Read the model definition and answer for the solid it produces. Units are mm, in the model's axes. Face numbers are marked on the shaded views. A direction names the side the tool comes from. Round coordinates to 2 decimals unless told otherwise and drop trailing zeros. Write each loop counter-clockwise with the first axis right and the second up, starting at its lowest first coordinate (ties: lowest second). Pieces come first, ordered by that corner, then holes. Notation, with made-up numbers: (43.5, 10.25) - (57.5, 10.25) arc R16 ccw to (57.5, 34.25) - close; hole circle Ø7 at (9, -5.75). An arc over 180 degrees is marked (long way). Answer as CSV lines item,"result". Start each with the question number.
1) Which of the six approach directions +Z, -Z, +X, -X, +Y, -Y give full straight-line access (tool end or side, diameter ignored) to the marked faces 1, 2 and 3?
2) Find section A-A on x = 9.5. Determine the outline of the cut face in (y, z).
3) For a pull along Y with two mould halves and no side action, classify the marked faces 4, 5, 6 and 7 as +Y half, -Y half, draft (parallel to the pull), parting line (faces both ways), or undercut.
4) Each of these flat-tipped pins is pushed along its axis until it touches: pin 1 (1.5 mm diameter, centred on y = -20.5, z = 6, fed in from -X); pin 2 (5 mm diameter, centred on x = 6, z = 4, fed in from -Y); pin 3 (5 mm diameter, centred on y = -37.5, z = 4.5, fed in from -X). Where does it stop, or does it pass through?
5) Find section B-B on z = 6.25. Determine the outline of the cut face in (x, y).
6) Find section D-D on y = -27.5. Determine the outline of the cut face in (x, z), then the cut area to 3 significant figures.
7) Consider line 1 along Y through (x, z) = (11, 2.25); line 2 along Y through (x, z) = (13, 7.25); line 3 along Y through (x, z) = (14.75, 2.75). Determine where each line is inside the solid, lowest interval first.
8) Find section C-C on x = 6.5. Determine the outline of the cut face in (y, z).
from build123d import *

# Parameters (mm, degrees)
F1_DEPTH = 10
F2_R     = 1
F3_SIZE  = 0.99999


# Not quite as in the source:
# - a fillet or chamfer is up to 0.001 mm smaller than in the source, because OpenCascade refuses the exact size


with BuildPart() as f1:
    # F0 (on Top) → F1 (new body)
    with BuildSketch(Plane.XY):
        Polygon((18, 0), (0, 0), (0, -3), (15, -3), (15, -13), (13, -15), (15, -17), (15, -37), (12, -37), (12, -34), (9, -34), (9, -40), (18, -40), align=None)
    extrude(amount=F1_DEPTH)

    # F2
    f2_edges = [f1.edges().sort_by_distance(p)[0] for p in [
        (13, -15, 5),
        (15, -13, 5),
        (15, -37, 5),
        (15, -17, 5),
        (15, -3, 5),
        (12, -37, 5),
    ]]
    fillet(f2_edges, radius=F2_R)

    # F3 (size 1 in the source; OpenCascade refuses exactly that, so slightly less here)
    f3_edges = [f1.edges().sort_by_distance(p)[0] for p in [
        (7, -3, 10),
        (14.707107, -3.292893, 10),
        (0, -1.5, 10),
        (15, -8.292893, 10),
        (9, 0, 10),
        (14.92388, -12.96847, 10),
        (18, -20, 10),
        (14.207107, -13.792893, 10),
        (13.5, -40, 10),
        (13.414214, -15, 10),
        (9, -37, 10),
        (14.207107, -16.207107, 10),
        (10.5, -34, 10),
        (14.92388, -17.03153, 10),
        (12, -35, 10),
        (15, -26.707107, 10),
        (12.292893, -36.707107, 10),
        (14.707107, -36.707107, 10),
        (13.5, -37, 10),
        (7, -3, 0),
        (14.707107, -3.292893, 0),
        (0, -1.5, 0),
        (15, -8.292893, 0),
        (9, 0, 0),
        (14.92388, -12.96847, 0),
        (18, -20, 0),
        (14.207107, -13.792893, 0),
        (13.5, -40, 0),
        (13.414214, -15, 0),
        (9, -37, 0),
        (14.207107, -16.207107, 0),
        (10.5, -34, 0),
        (14.92388, -17.03153, 0),
        (12, -35, 0),
        (15, -26.707107, 0),
        (12.292893, -36.707107, 0),
        (14.707107, -36.707107, 0),
        (13.5, -37, 0),
    ]]
    chamfer(f3_edges, length=F3_SIZE)


solid = f1.part
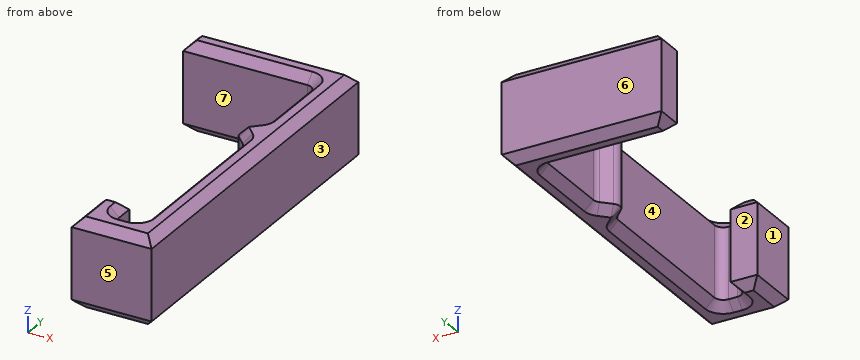
Check values:
1,face 1,"+Z, -Z, -X, -Y"
1,face 2,"+Z, -Z, -X"
1,face 3,"+Z, -Z, +X, +Y, -Y"
2,outline,"(-40, 1) - (-39.5, 0.5) - (-34.5, 0.5) - (-34, 1) - (-34, 9) - (-34.5, 9.5) - (-39.5, 9.5) - (-40, 9) - close; (-3, 1) - (-2, 0) - (-1, 0) - (0, 1) - (0, 9) - (-1, 10) - (-2, 10) - (-3, 9) - close"
3,face 4,"undercut"
3,face 5,"-Y half"
3,face 6,"+Y half"
3,face 7,"undercut"
4,pin 1,"stops at x = 15"
4,pin 2,"stops at y = -3"
4,pin 3,"stops at x = 9"
5,outline,"(0, -3) - (14, -3) arc R1 cw to (15, -4) - (15, -12.59) arc R1 cw to (14.71, -13.29) - (13.71, -14.29) arc R1 ccw to (13.71, -15.71) - (14.71, -16.71) arc R1 cw to (15, -17.41) - (15, -36) arc R1 cw to (14, -37) - (13, -37) arc R1 cw to (12, -36) - (12, -34) - (9, -34) - (9, -40) - (18, -40) - (18, 0) - (0, 0) - close"
6,outline,"(15, 1) - (16, 0) - (17, 0) - (18, 1) - (18, 9) - (17, 10) - (16, 10) - (15, 9) - close"
6,area,"28.0 mm^2"
7,line 1,"y = -40 to -34, -3 to 0"
7,line 2,"y = -40 to -37, -3 to 0"
7,line 3,"y = -40 to -36.66, -16.75 to -13.25, -3.34 to 0"
8,outline,"(-3, 1) - (-2, 0) - (-1, 0) - (0, 1) - (0, 9) - (-1, 10) - (-2, 10) - (-3, 9) - close"
